Model file for the job. Use its own axes, mm. Face numbers are marked on the shaded views. A direction names the side the tool comes from. Round coordinates to 2 decimals unless told otherwise and drop trailing zeros. Order: outer loops, then holes, each group sorted by start corner. A loop starts at its lowest first (then second) coordinate and runs counter-clockwise, first axis right, second up. Notation, with made-up numbers: (63.25, -30) -> (90.25, -30) arc R26 cw to (90.25, 4) -> close; hole circle Ø6 at (-2, 41.5). An arc over 180 degrees is marked (long way). Use CSV: the item, a comma, the result in double quotes.
```python
from build123d import *

# Parameters (mm, degrees)
EXTRUDE_1_DEPTH          = 42.3
EXTRUDE_START            = 3
EXTRUDE_2_DEPTH          = 3
SKETCH_3_W               = 37.077621282
SKETCH_3_H               = 5
EXTRUDE_4_DEPTH          = 20
SKETCH_5_W               = 37.077621282
SKETCH_5_H               = 5
EXTRUDE_5_DEPTH          = 20
CUT_EXTRUDE_1_REACH      = 102.493
SKETCH_6_R               = 5
CUT_EXTRUDE_2_REACH      = 102.493
SKETCH_7_R               = 5
CUT_EXTRUDE_3_DEPTH      = 137.919145849
CUT_EXTRUDE_3_DEPTH_BACK = 137.919145849
SKETCH_9_W               = 62.954996742
SKETCH_9_H               = 12


with BuildPart() as part:
    # Sketch 1 → Extrude 1 (new body)
    with BuildSketch(Plane(origin=(0, 0, 0), x_dir=(1, 0, 0), z_dir=(0, 1, 0))):
        with BuildLine():
            Line((-51.25, 18.538810641), (-51.25, -18.538810641))
            ThreePointArc((-51.25, -18.538810641), (0, -54.5), (51.25, -18.538810641))
            Line((51.25, -18.538810641), (51.25, 18.538810641))
            ThreePointArc((51.25, 18.538810641), (0, 54.5), (-51.25, 18.538810641))
        make_face()
        with BuildLine():
            Line((-46.25, 17.640507362), (-46.25, -17.640507362))
            ThreePointArc((-46.25, -17.640507362), (0, -49.5), (46.25, -17.640507362))
            Line((46.25, -17.640507362), (46.25, 17.640507362))
            ThreePointArc((46.25, 17.640507362), (0, 49.5), (-46.25, 17.640507362))
        make_face(mode=Mode.SUBTRACT)
    extrude(amount=EXTRUDE_1_DEPTH)

    # Sketch 2 → Extrude 2 (add)
    with BuildSketch(Plane(origin=(0, 0, 0), x_dir=(-1, 0, 0), z_dir=(0, -1, 0)).offset(EXTRUDE_START)):
        with BuildLine():
            Line((51.25, -18.538810641), (51.25, 18.538810641))
            ThreePointArc((51.25, 18.538810641), (0, 54.5), (-51.25, 18.538810641))
            Line((-51.25, 18.538810641), (-51.25, -18.538810641))
            ThreePointArc((-51.25, -18.538810641), (0, -54.5), (51.25, -18.538810641))
        make_face()
    extrude(amount=-EXTRUDE_2_DEPTH)

    # Sketch 3 → Extrude 4 (add)
    with BuildSketch(Plane.ZY.offset(51.25)):
        with Locations((0, 39.8)):
            Rectangle(SKETCH_3_W, SKETCH_3_H)
    extrude(amount=EXTRUDE_4_DEPTH)

    # Sketch 5 → Extrude 5 (add)
    with BuildSketch(Plane(origin=(51.25, 0, 0), x_dir=(0, 0, -1), z_dir=(1, 0, 0))):
        with Locations((0, 39.8)):
            Rectangle(SKETCH_5_W, SKETCH_5_H)
    extrude(amount=EXTRUDE_5_DEPTH)

    # Sketch 6 → Cut-Extrude 1 (cut, up to next)
    with BuildSketch(Plane(origin=(0, 42.3, 0), x_dir=(1, 0, 0), z_dir=(0, 1, 0)), mode=Mode.PRIVATE) as cut_extrude_1_sk1:
        with Locations(Location((-61.25, 0, 0), (0, 0, 270))):
            Circle(SKETCH_6_R)
    cut_extrude_1_tool1 = extrude(cut_extrude_1_sk1.sketch, amount=-CUT_EXTRUDE_1_REACH, mode=Mode.PRIVATE) & part.part
    add(cut_extrude_1_tool1.solids().sort_by_distance((-61.25, 42.3, 0))[0], mode=Mode.SUBTRACT)

    # Sketch 7 → Cut-Extrude 2 (cut, up to next)
    with BuildSketch(Plane(origin=(0, 42.3, 0), x_dir=(1, 0, 0), z_dir=(0, 1, 0)), mode=Mode.PRIVATE) as cut_extrude_2_sk1:
        with Locations(Location((61.25, 0, 0), (0, 0, 270))):
            Circle(SKETCH_7_R)
    cut_extrude_2_tool1 = extrude(cut_extrude_2_sk1.sketch, amount=-CUT_EXTRUDE_2_REACH, mode=Mode.PRIVATE) & part.part
    add(cut_extrude_2_tool1.solids().sort_by_distance((61.25, 42.3, 0))[0], mode=Mode.SUBTRACT)

    # Sketch 9 → Cut-Extrude 3 (cut, two sides: drawn at the far end of the back side and taken through both)
    with BuildSketch(Plane(origin=(0, 0, -54.5), x_dir=(-1, 0, 0), z_dir=(0, 0, -1)).offset(-CUT_EXTRUDE_3_DEPTH_BACK)):
        with Locations((0, 7)):
            Rectangle(SKETCH_9_W, SKETCH_9_H)
    extrude(amount=CUT_EXTRUDE_3_DEPTH + CUT_EXTRUDE_3_DEPTH_BACK, mode=Mode.SUBTRACT)


solid = part.part
```
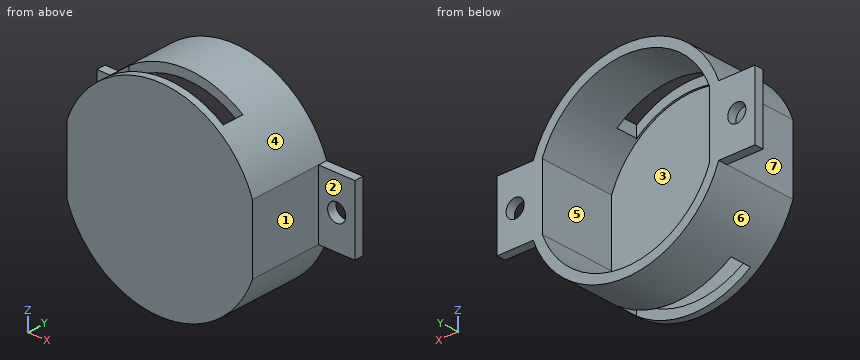
Q1. Cut at B-B (x = 61.25). Give the cut face in (y, z), plus the area to 3 significant figures.
From the geometry:
outline,"(37.3, -18.54) -> (42.3, -18.54) -> (42.3, -5) -> (37.3, -5) -> close; (37.3, 5) -> (42.3, 5) -> (42.3, 18.54) -> (37.3, 18.54) -> close"
area,"135 mm²"
Q2. Which spindle directions (+Z, -Z, +X, -X, +Y, -Y) get a long thin tool onto all of the face, cutting with end or side? Do the marked faces 5, 6 and 7. Say none if no direction does.
From the geometry:
face 5,"+Y"
face 6,"-Z, +Y, -Y"
face 7,"+Z, -Z, -X, -Y"
Q3. Mould opens along X. For the marked faces 1, 2, 3 and 4 say: +X half, -X half, draft (parallel to the pull), parting line (faces both ways), or undercut.
From the geometry:
face 1,"+X half"
face 2,"draft"
face 3,"undercut"
face 4,"parting line"
Q4. Probe line 1 along X through (y, z) = (39.15, 0); line 2 along X through (y, z) = (17.5, -16.5); line 3 along Z through (x, y) = (-61, 39). List the from-to ranges inside material, lowest first.
From the geometry:
line 1,"x = -71.25 to -66.25, -56.25 to -46.25, 46.25 to 56.25, 66.25 to 71.25"
line 2,"x = -51.25 to -46.25, 46.25 to 51.25"
line 3,"z = -18.54 to -4.99, 4.99 to 18.54"
Q5. Pin check, flat tips, straight feed: pin 1 (2.5 mm diameter, centred on x = 59.5, y = 39.5, fed in from -Z); pin 2 (5.5 mm diameter, centred on x = 65.5, y = 39, fed in from +Z); pin 3 (16 mm diameter, centred on x = 61.5, z = -6, fed in from -Y); pin 4 (12 mm diameter, centred on x = 46, z = 32.5, fed in from -Y). Stop position of each tip, or through.
From the geometry:
pin 1,"stops at z = -18.54"
pin 2,"stops at z = 18.54"
pin 3,"stops at y = 37.3"
pin 4,"stops at y = -3"
Q6. Cut at D-D (x = -0.5). Give the cut face in (y, z).
From the geometry:
outline,"(-3, -54.5) -> (1, -54.5) -> (1, -49.5) -> (0, -49.5) -> (0, 49.5) -> (1, 49.5) -> (1, 54.5) -> (-3, 54.5) -> close; (13, -54.5) -> (42.3, -54.5) -> (42.3, -49.5) -> (13, -49.5) -> close; (13, 49.5) -> (42.3, 49.5) -> (42.3, 54.5) -> (13, 54.5) -> close"
Q7. Cut at C-C (y = 35.5). Give the cut face in (x, z), plus the area to 3 significant figures.
From the geometry:
outline,"(-51.25, -18.54) arc R54.5 ccw to (51.25, -18.54) -> (51.25, 18.54) arc R54.5 ccw to (-51.25, 18.54) -> close; hole (-46.25, -17.64) arc R49.5 ccw to (46.25, -17.64) -> (46.25, 17.64) arc R49.5 ccw to (-46.25, 17.64) -> close"
area,"1,630 mm²"
Q8. Cut at A-A (y = 6.5). Give the cut face in (x, z), plus the area to 3 significant figures.
From the geometry:
outline,"(-51.25, -18.54) arc R54.5 ccw to (-31.48, -44.49) -> (-31.48, -38.2) arc R49.5 cw to (-46.25, -17.64) -> (-46.25, 17.64) arc R49.5 cw to (-31.48, 38.2) -> (-31.48, 44.49) arc R54.5 ccw to (-51.25, 18.54) -> close; (31.48, -44.49) arc R54.5 ccw to (51.25, -18.54) -> (51.25, 18.54) arc R54.5 ccw to (31.48, 44.49) -> (31.48, 38.2) arc R49.5 cw to (46.25, 17.64) -> (46.25, -17.64) arc R49.5 cw to (31.48, -38.2) -> close"
area,"950 mm²"
